from build123d import *

# Parameters (mm, degrees)
ESBO_O1_W                = 50
ESBO_O1_H                = 12
ESBO_O1_R                = 1.75
RESSALTO_EXTRUS_O1_DEPTH = 2


with BuildPart() as part:
    # Esboço1 → Ressalto-extrusão1 (new body)
    with BuildSketch(Plane(origin=(0, 0, 0), x_dir=(1, 0, 0), z_dir=(0, 1, 0))):
        Rectangle(ESBO_O1_W, ESBO_O1_H)
        with Locations(Location((-15, 0, 0), (0, 0, 270))):
            Circle(ESBO_O1_R, mode=Mode.SUBTRACT)
        with Locations(Location((15, 0, 0), (0, 0, 270))):
            Circle(ESBO_O1_R, mode=Mode.SUBTRACT)
    extrude(amount=RESSALTO_EXTRUS_O1_DEPTH)


solid = part.part
Source: CAD feature listing. Evaluate the final solid. Frame: model axes, mm. Coordinates: 2 decimals unless noted, no trailing zeros. Order: outer loops, then holes, each group sorted by start corner. A loop starts at its lowest first (then second) coordinate and runs counter-clockwise, first axis right, second up. Notation, with made-up numbers: M 36,-21 L 53,-21 A7 ccw 53,-16 Z; hole C -33.75,-25 d3. An arc over 180 degrees is marked long. Write each question's results on one line, items separated by ' | '. Start each with the question number.
Item 1: Draft query along X for faces 1 (the face through (-13.265, 0.986, -0.228)), 2 (the face through (16.735, 0.986, -0.228)), 3 (the face through (0, 1, -6)), 4 (the face through (-25, 1, 0)). Return one class per face: pulls with the +X half, pulls with the -X half, needs draft (parallel to the pull), parting line crosses it, or undercut.
Item 2: First-contact query: pin 1 Ø3 at (x, z) = (-15, 0) entering from -Y. Flat tip, straight axial feed; report the tip coordinate or a pass-through.
Item 3: Line query: probe 1 along X at (y, z) = (1.6, 0); probe 2 along X at (y, z) = (0.95, 1.5); probe 3 along Z at (x, y) = (15.5, 0.1). Output: solid intervals per line, ascending.
Item 4: Cut plane A-A (x = -15). Return loops of the section in (y, z).
Item 5: Cut plane B-B (z = 0). Return loops of the section in (x, y), and give its area (3 significant figures).
Item 6: Cut plane C-C (y = 1.6). Return loops of the section in (x, z), and give its area (3 significant figures).
Checked values:
1) face 1: undercut | face 2: undercut | face 3: needs draft | face 4: pulls with the -X half
2) pin 1: passes through
3) probe 1: x = -25 to -16.75, -13.25 to 13.25, 16.75 to 25 | probe 2: x = -25 to -15.9, -14.1 to 14.1, 15.9 to 25 | probe 3: z = -6 to -1.68, 1.68 to 6
4) outline: M 0,-6 L 2,-6 L 2,-1.75 L 0,-1.75 Z; M 0,1.75 L 2,1.75 L 2,6 L 0,6 Z
5) outline: M -25,0 L -16.75,0 L -16.75,2 L -25,2 Z; M -13.25,0 L 13.25,0 L 13.25,2 L -13.25,2 Z; M 16.75,0 L 25,0 L 25,2 L 16.75,2 Z | area: 86.0 mm2
6) outline: M -25,-6 L 25,-6 L 25,6 L -25,6 Z; hole C -15,0 d3.5; hole C 15,0 d3.5 | area: 581 mm2
